Part print with two shaded views. Sizes in mm from the minimum x, y, z corner. A direction names the side the tool comes from. Give positions to 0.01 mm unless a question says otherwise; leave off trailing zeros. Order: outer loops, then holes, each group sorted by start corner. A loop starts at its lowest first (then second) coordinate and runs counter-clockwise, first axis right, second up. Notation, with made-up numbers: M -13.75,-15.5 L 13.25,-15.5 A23 ccw 13.25,15.5 Z; hole C 27,-3.75 d4. An arc over 180 degrees is marked long. Return JSON: item names as keys, results as strings.
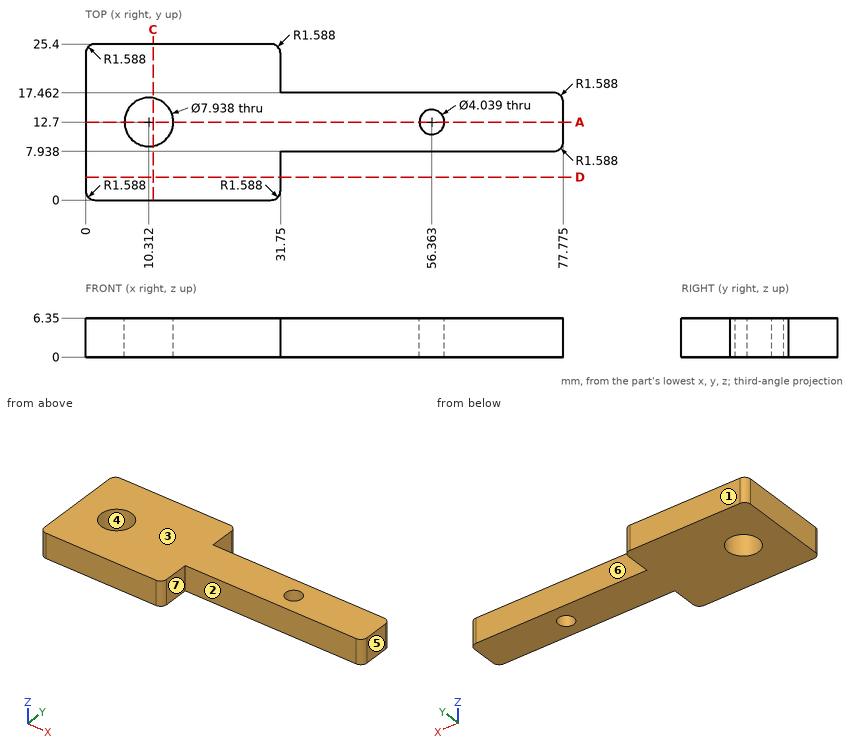
Q1. Pin check, flat tips, straight feed: pin 1 (6 mm diameter, centred on x = 36, y = 11, fed in from -Z); pin 2 (3 mm diameter, centred on y = 5, z = 3, fed in from +X). Stop position of each tip, or through.
Established:
{"pin 1": "stops at z = 0", "pin 2": "stops at x = 31.75"}
Q2. Band-saw the part on D-D (y = 3.75). Give the cut face in (x, z), then the cut area to 3 significant figures.
Established:
{"outline": "M 0,0 L 31.75,0 L 31.75,6.35 L 0,6.35 Z", "area": "202 mm²"}
Q3. 3-axis set-ups, long thin cutter, end or side, ignore diameter. For the marked faces 5, 6 and 7: which of +Z, -Z, +X, -X, +Y, -Y reach the whole face in a straight line?
Established:
{"face 5": "+Z, -Z, +X, +Y, -Y", "face 6": "+Z, -Z, +X, +Y", "face 7": "+Z, -Z, +X, -Y"}
Q4. Band-saw the part on A-A (y = 12.7). Give the number of separate pieces and of enclosed holes in the cut face, then the cut area to 3 significant figures.
Established:
{"separate pieces": "3", "enclosed holes": "0", "area": "418 mm²"}
Q5. Probe line 1 along X through (y, z) = (13.75, 4) (1 decimal); line 2 along Y through (x, z) = (60, 3.5); line 3 along X through (y, z) = (5.25, 5.5). List the from-to ranges inside material, lowest first.
Established:
{"line 1": "x = 0 to 6.5, 14.1 to 54.6, 58.1 to 77.8", "line 2": "y = 7.94 to 17.46", "line 3": "x = 0 to 31.75"}
Q6. Two-plate mould, pull along Y, no slides. Class the marked faces 1, 2, 3 and 4: +Y half, -Y half, draft (parallel to the pull), parting line (faces both ways), or undercut.
Established:
{"face 1": "+Y half", "face 2": "-Y half", "face 3": "draft", "face 4": "undercut"}
Q7. Band-saw the part on C-C (x = 11). Give the cut face in (y, z).
Established:
{"outline": "M 0,0 L 8.79,0 L 8.79,6.35 L 0,6.35 Z; M 16.61,0 L 25.4,0 L 25.4,6.35 L 16.61,6.35 Z"}
